Verification items for this drawing (mm, ordinates from the low corner). Round coordinates to 2 decimals unless told otherwise and drop trailing zeros. Order: outer loops, then holes, each group sorted by start corner. A loop starts at its lowest first (then second) coordinate and runs counter-clockwise, first axis right, second up. Notation, with made-up numbers: (22, -21.75) -> (63, -21.75) arc R36 ccw to (63, 15.25) -> close; hole circle Ø6 at (64, 71.25). An arc over 180 degrees is marked (long way). Answer in a Markdown table with one row per item.
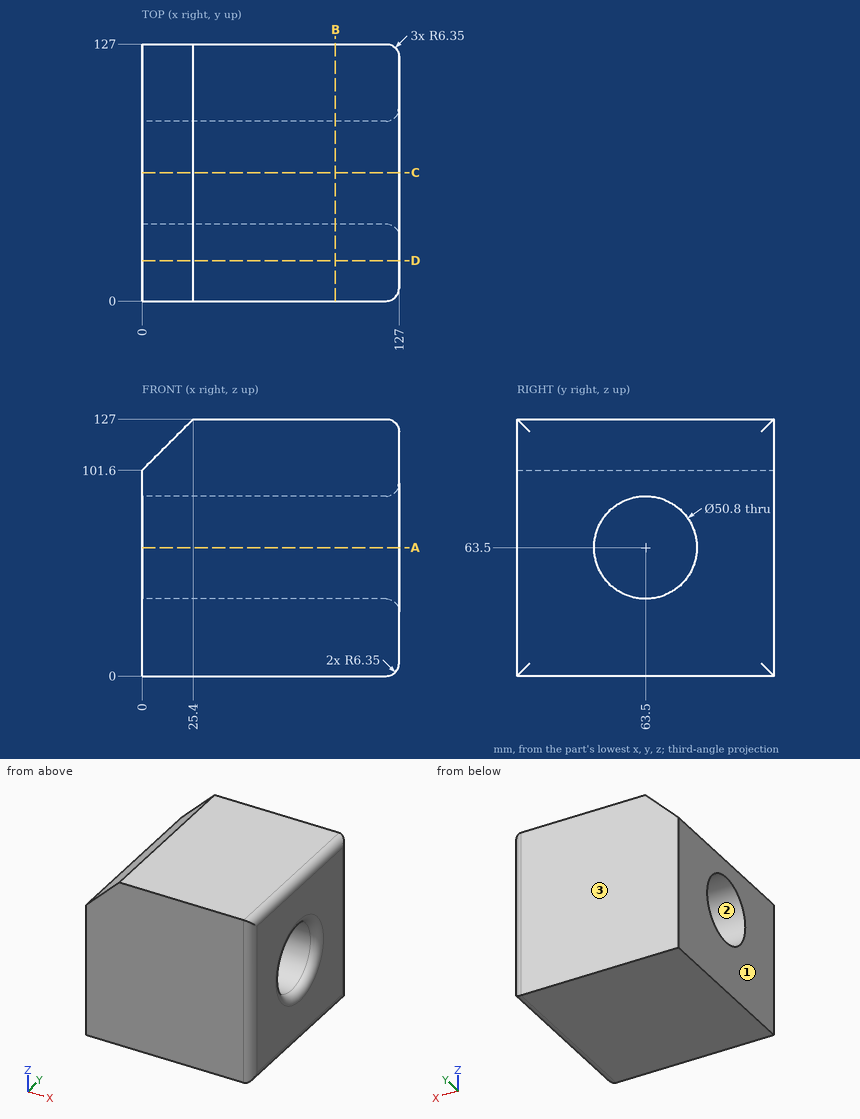
Item 1: Cross-section at A-A (z = 63.5). Record the boundary of the cut face in (x, y), and give its area (3 significant figures).
Result sheet:
| item | result |
|---|---|
| outline | (0, 0) -> (120.65, 0) arc R6.35 ccw to (127, 6.35) -> (127, 31.75) arc R6.35 ccw to (120.65, 38.1) -> (0, 38.1) -> close; (0, 88.9) -> (120.65, 88.9) arc R6.35 ccw to (127, 95.25) -> (127, 120.65) arc R6.35 ccw to (120.65, 127) -> (0, 127) -> close |
| area | 9,640 mm^2 |
Item 2: Mould release check, pull along Y, two halves, no side actions. Record for the marked faces 1, 2 and 3: pulls with the +Y half, pulls with the -Y half, needs draft (parallel to the pull), parting line crosses it, or undercut.
Result sheet:
| item | result |
|---|---|
| face 1 | needs draft |
| face 2 | undercut |
| face 3 | pulls with the +Y half |
Item 3: Depth check by flat-ended pin: P1, Ø1.5, axis at y = 91, z = 104, coming from the -X side. Enter the tip coordinate at first touch or a pass-through.
Result sheet:
| item | result |
|---|---|
| P1 | stops at x = 1.65 |
Item 4: Cross-section at C-C (y = 63.5). Record the boundary of the cut face in (x, z).
Result sheet:
| item | result |
|---|---|
| outline | (0, 0) -> (120.65, 0) arc R6.35 ccw to (127, 6.35) -> (127, 31.75) arc R6.35 ccw to (120.65, 38.1) -> (0, 38.1) -> close; (0, 88.9) -> (120.65, 88.9) arc R6.35 ccw to (127, 95.25) -> (127, 120.65) arc R6.35 ccw to (120.65, 127) -> (25.4, 127) -> (0, 101.6) -> close |
Item 5: Cross-section at B-B (x = 95.5). Record the boundary of the cut face in (y, z), and give its area (3 significant figures).
Result sheet:
| item | result |
|---|---|
| outline | (0, 0) -> (127, 0) -> (127, 127) -> (0, 127) -> close; hole circle Ø50.8 at (63.5, 63.5) |
| area | 14,100 mm^2 |
Item 6: Scan lines: line 1 (Z direction, x = 49, y = 63.5); line 2 (Y direction, x = 57, z = 50.5). Record each from-to range of solid material in increasing order. Write a range as [from, to].
Result sheet:
| item | result |
|---|---|
| line 1 | z = [0, 38.1], [88.9, 127] |
| line 2 | y = [0, 41.68], [85.32, 127] |
Item 7: Cross-section at D-D (y = 20). Record the boundary of the cut face in (x, z), and give its area (3 significant figures).
Result sheet:
| item | result |
|---|---|
| outline | (0, 0) -> (120.65, 0) arc R6.35 ccw to (127, 6.35) -> (127, 120.65) arc R6.35 ccw to (120.65, 127) -> (25.4, 127) -> (0, 101.6) -> close |
| area | 15,800 mm^2 |
